Print and shaded views of the part. All mm, measured from the part's lowest x, y and z. A direction names the side the tool comes from. Coordinates: 2 decimals unless noted, no trailing zeros. Loops run counter-clockwise (first coordinate to the right, second up) from the corner with the lowest first, then second, coordinate; pieces in that order, holes last. Notation, with made-up numbers: M 81,72 L 103,72 A16 ccw 103,78 Z; hole C 78,16 d2. An arc over 180 degrees is marked long. One line per question, with ' | ' between items. Start each with the question number.
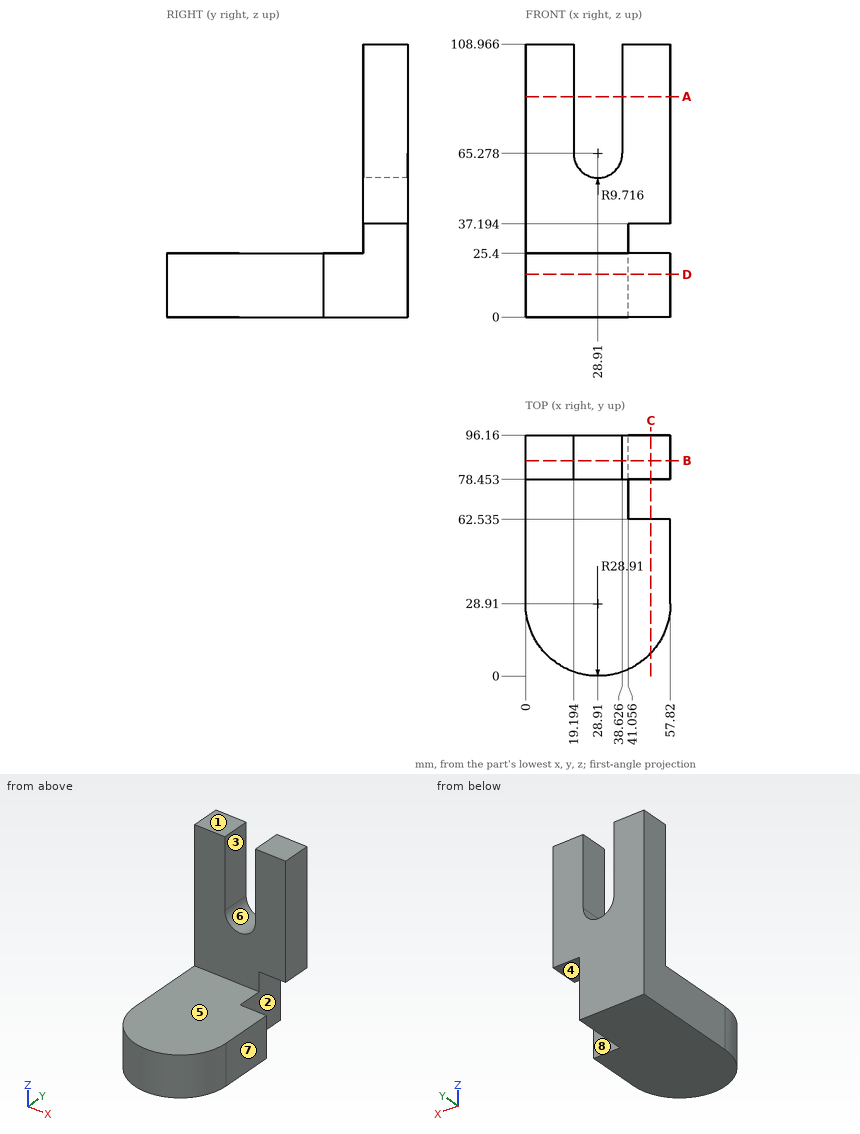
(1) Drill centre lines: line 1 (X direction, y = 88.5, z = 75); line 2 (Y direction, x = 40, z = 89); line 3 (Z direction, x = 7, y = 13.5). Where is each one in solid material? Low to high. Write a range as [from, to].
(2) Two-plate mould, pull along X, no slides. Class the marked faces 6, 7 and 8: pulls with the +X half, pulls with the -X half, needs draft (parallel to the pull), parting line crosses it, or undercut.
(3) Band-saw the part on A-A on z = 88. Write the cut outline in (x, y), then the cut area to 3 significant figures.
(4) Band-saw the part on C-C on x = 50. Write the cut outline in (y, z) (1 decimal), then the cut area to 3 significant figures.
(5) Band-saw the part on B-B on y = 86. Write the cut outline in (x, z).
(6) Band-saw the part on D-D on z = 17. Write the cut outline in (x, y) (1 decimal), then the cut area to 3 significant figures.
(7) 3-axis set-ups, long thin cutter, end or side, ignore diameter. For the marked faces 1, 2, 3, 4 and 5: which of +Z, -Z, +X, -X, +Y, -Y reach the whole face in a straight line?
(8) Pin check, flat tips, straight feed: P1, Ø17.5, axis at x = 27, z = 56, coming from the -Y side; P2, Ø8.5, axis at x = 52, z = 14, coming from the +Y side (1 decimal); P3, Ø5, axis at x = 53.5, y = 88, coming from the -Z side. Stop position of each tip, or through.
Computed values:
1) line 1: [0, 19.19], [38.63, 57.82] | line 2: [78.45, 96.16] | line 3: [0, 25.4]
2) face 6: undercut | face 7: pulls with the +X half | face 8: needs draft
3) outline: M 0,78.45 L 19.19,78.45 L 19.19,96.16 L 0,96.16 Z; M 38.63,78.45 L 57.82,78.45 L 57.82,96.16 L 38.63,96.16 Z | area: 680 mm^2
4) outline: M 9.1,0 L 62.5,0 L 62.5,25.4 L 9.1,25.4 Z; M 78.5,37.2 L 96.2,37.2 L 96.2,109 L 78.5,109 Z | area: 2,630 mm^2
5) outline: M 0,0 L 41.06,0 L 41.06,37.19 L 57.82,37.19 L 57.82,108.97 L 38.63,108.97 L 38.63,65.28 A9.72 cw 19.19,65.28 L 19.19,108.97 L 0,108.97 Z
6) outline: M 0,28.9 A28.9 ccw 57.8,28.9 L 57.8,62.5 L 41.1,62.5 L 41.1,96.2 L 0,96.2 Z | area: 4,640 mm^2
7) face 1: +Z, +X, -X, +Y, -Y | face 2: -Z, +X, +Y | face 3: +Z, +Y, -Y | face 4: -Z, +X, +Y, -Y | face 5: +Z, +X, -X, -Y
8) P1: y = 78.45 | P2: y = 62.5 | P3: z = 37.19
